For this review, use the dimensioned drawing (mm, ordinates from the lowest corner) and the shaded views. A direction names the side the tool comes from. Round coordinates to 2 decimals unless told otherwise and drop trailing zeros. Loops run counter-clockwise (first coordinate to the right, second up) from the corner with the lowest first, then second, coordinate; pieces in that order, holes last. Notation, with made-up numbers: (57, 20.5) -> (61, 20.5) arc R15 ccw to (61, 29.5) -> close; hole circle Ø9 at (89, 0.25). An arc over 180 degrees is marked (long way). Write each question's results on one line, items separated by ' | '. Start each with the question number.
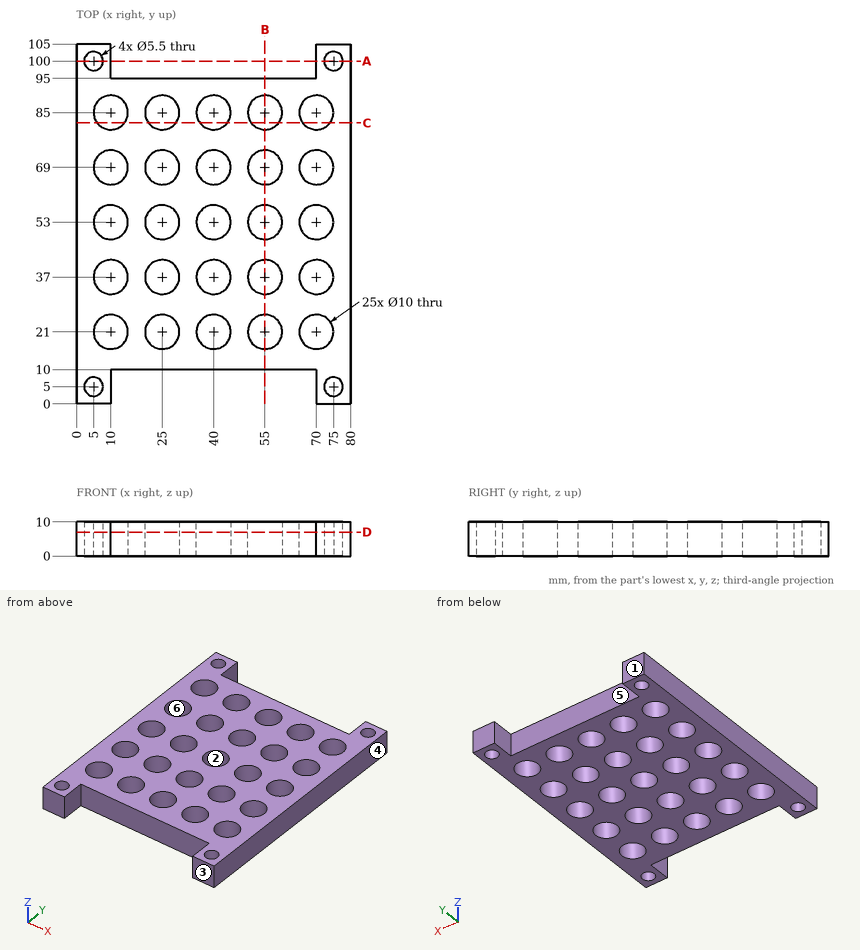
1) Take a section at C-C (y = 82). Write out the cut boundary in (x, z), plus the area to 3 significant figures.
2) To check wall thickness, follow line 1 (Y direction, x = 25, z = 7.25); line 2 (X direction, y = 51.5, z = 9.5); line 3 (Y direction, x = 56, z = 5.25). State the ranges of each line that lie inside material, in increasing order. Write a range as from..to.
3) Take a section at A-A (y = 100). Write out the cut boundary in (x, z), plus the area to 3 significant figures.
4) Take a section at B-B (x = 55). Write out the cut boundary in (y, z), plus the area to 3 significant figures.
5) Take a section at D-D (z = 7). State how many separate pieces and enclosed holes the cut face has, plus the area to 3 significant figures.
6) Insertion check: pin 1 (2 mm diameter, centred on y = 44.5, z = 7.5, fed in from -X); pin 2 (2 mm diameter, centred on x = 31, z = 9, fed in from -Y). Each pin has a flat end and moves straight along its axis. Give the tip position at first contact, or say it passes through.
7) For the marked faces 5 and 6, list the 3-axis set-ups (+Z, -Z, +X, -X, +Y, -Y) from which the entire face can be reached by the end or side of a thin tool; tool diameter is ignored.
8) The part is to be moulded in two halves that separate along Y. For the marked faces 1, 2, 3 and 4, say which applies: +Y half, -Y half, draft (parallel to the pull), parting line (faces both ways), or undercut.
Geometry check:
1) outline: (0, 0) -> (6, 0) -> (6, 10) -> (0, 10) -> close; (14, 0) -> (21, 0) -> (21, 10) -> (14, 10) -> close; (29, 0) -> (36, 0) -> (36, 10) -> (29, 10) -> close; (44, 0) -> (51, 0) -> (51, 10) -> (44, 10) -> close; (59, 0) -> (66, 0) -> (66, 10) -> (59, 10) -> close; (74, 0) -> (80, 0) -> (80, 10) -> (74, 10) -> close | area: 400 mm^2
2) line 1: y = 10..16, 26..32, 42..48, 58..64, 74..80, 90..95 | line 2: x = 0..5.23, 14.77..20.23, 29.77..35.23, 44.77..50.23, 59.77..65.23, 74.77..80 | line 3: y = 10..16.1, 25.9..32.1, 41.9..48.1, 57.9..64.1, 73.9..80.1, 89.9..95
3) outline: (0, 0) -> (2.25, 0) -> (2.25, 10) -> (0, 10) -> close; (7.75, 0) -> (10, 0) -> (10, 10) -> (7.75, 10) -> close; (70, 0) -> (72.25, 0) -> (72.25, 10) -> (70, 10) -> close; (77.75, 0) -> (80, 0) -> (80, 10) -> (77.75, 10) -> close | area: 90.0 mm^2
4) outline: (10, 0) -> (16, 0) -> (16, 10) -> (10, 10) -> close; (26, 0) -> (32, 0) -> (32, 10) -> (26, 10) -> close; (42, 0) -> (48, 0) -> (48, 10) -> (42, 10) -> close; (58, 0) -> (64, 0) -> (64, 10) -> (58, 10) -> close; (74, 0) -> (80, 0) -> (80, 10) -> (74, 10) -> close; (90, 0) -> (95, 0) -> (95, 10) -> (90, 10) -> close | area: 350 mm^2
5) separate pieces: 1 | enclosed holes: 29 | area: 5,140 mm^2
6) pin 1: stops at x = 0 | pin 2: stops at y = 10
7) face 5: +Z, -Z, +Y | face 6: +Z, -Z
8) face 1: +Y half | face 2: undercut | face 3: -Y half | face 4: draft
